Here's how the part is built. I have some questions about the finished solid (model axes, mm). A direction names the side the tool comes from. Coordinates: 2 decimals unless noted, no trailing zeros. Write each loop counter-clockwise with the first axis right and the second up, starting at its lowest first coordinate (ties: lowest second). Pieces come first, ordered by that corner, then holes.
```python
from build123d import *

# Parameters (mm, degrees)
CROQUIS1_W              = 66.05
CROQUIS1_H              = 54.82
SALIENTE_EXTRUIR1_DEPTH = 1.72


with BuildPart() as part:
    # Croquis1 → Saliente-Extruir1 (new body)
    with BuildSketch(Plane(origin=(0, 0, 0), x_dir=(1, 0, 0), z_dir=(0, 1, 0))):
        Rectangle(CROQUIS1_W, CROQUIS1_H)
        Polygon((35.675, 10.59), (33.025, 13.09), (33.025, -24.91), (35.675, -22.11), align=None)
    extrude(amount=SALIENTE_EXTRUIR1_DEPTH)


solid = part.part
```
1) On a 3-axis mill with a long thin cutter (end or side, diameter ignored), from which of +Z, -Z, +X, -X, +Y, -Y can I reach the whole of each face in a straight line? I mean faces 1 (the face through (33.025, 1, -20)), 2 (the face through (1, 0, 0)), 3 (the face through (33.025, 1, 26)). Say none if no direction works.
Values follow:
face 1: -Z, +X, +Y, -Y
face 2: +Z, -Z, +X, -X, -Y
face 3: +Z, +X, +Y, -Y
2) Imagine slicing it at A-A on z = -21. Please give me the cut outline in (x, y) (3 decimals).
Values follow:
outline: (-33.025, 0) - (33.025, 0) - (33.025, 1.72) - (-33.025, 1.72) - close
3) I need wall thicknesses on probe 1 along X at (y, z) = (1.55, -18) (3 decimals). Which ranges of the line are inside material? Lowest first, please.
Values follow:
probe 1: x = -33.025 to 33.025
4) Will this pin go through, and if not, where does the flat tip stop? pin 1 (4 mm diameter, centred on x = 5.5, z = -3.5, fed in from -Y).
Values follow:
pin 1: stops at y = 0
